from build123d import *

# Parameters (mm, degrees)
F0_R     = 15.24
F0_R_2   = 12.7
F0_R_3   = 11.43
F1_DEPTH = 19.05
F0_R_4   = 1.27
F0_R_5   = 4.8718647292
F2_DEPTH = 12.7
F3_DEPTH = 6.35
F5_DEPTH = 7.62


# Not quite as in the source:
# - a feature of the source that left no trace in its solid (it failed there, or was rolled back) is left out
# - the program builds the solid bodies; features that only make, move or delete a surface that nothing else refers to are left out


with BuildPart() as f1:
    # F0 (on Front) → F1 (new body)
    with BuildSketch(Plane.XZ):
        Circle(F0_R)
        Circle(F0_R_2, mode=Mode.SUBTRACT)
        Circle(F0_R_2)
        Circle(F0_R_3, mode=Mode.SUBTRACT)
    extrude(amount=F1_DEPTH)

    # F0 (on Front) → F2 (join)
    with BuildSketch(Plane.XZ):
        Circle(F0_R_3)
        with Locations((-6.35, -3.6661742094)):
            Circle(F0_R_4, mode=Mode.SUBTRACT)
        with Locations((0, -7.3323484187)):
            Circle(F0_R_4, mode=Mode.SUBTRACT)
        with Locations((6.35, -3.6661742094)):
            Circle(F0_R_4, mode=Mode.SUBTRACT)
        with Locations((-6.35, 3.6661742094)):
            Circle(F0_R_4, mode=Mode.SUBTRACT)
        Circle(F0_R_5, mode=Mode.SUBTRACT)
        with Locations((6.35, 3.6661742094)):
            Circle(F0_R_4, mode=Mode.SUBTRACT)
        with Locations((0, 7.3323484187)):
            Circle(F0_R_4, mode=Mode.SUBTRACT)
    extrude(amount=F2_DEPTH)

    # F0 (on Front) → F3 (join)
    with BuildSketch(Plane.XZ):
        Circle(F0_R_5)
        Polygon((3.175, 1.27), (3.175, -1.27), (1.27, -1.27), (1.27, -3.175), (-1.27, -3.175), (-1.27, -1.27), (-3.175, -1.27), (-3.175, 1.27), (-1.27, 1.27), (-1.27, 3.175), (1.27, 3.175), (1.27, 1.27), align=None, mode=Mode.SUBTRACT)
        with Locations((6.35, 3.6661742094)):
            Circle(F0_R_4)
    extrude(amount=F3_DEPTH)

    # F0 (on Front) + F4 (on face) → F5 (join)
    with BuildSketch(Plane.XZ):
        with Locations((0, 7.3323484187)):
            Circle(F0_R_4)
        with Locations((6.35, -3.6661742094)):
            Circle(F0_R_4)
        with Locations((0, -7.3323484187)):
            Circle(F0_R_4)
        with Locations((-6.35, -3.6661742094)):
            Circle(F0_R_4)
        with Locations((-6.35, 3.6661742094)):
            Circle(F0_R_4)
    with BuildSketch(Plane(origin=(0, 0, 0), x_dir=(-1, 0, 0), z_dir=(0, 1, 0))):
        with BuildLine():
            ThreePointArc((-1.27, 7.3323484187), (0, 6.0623484187), (1.27, 7.3323484187))
            ThreePointArc((1.27, 7.3323484187), (0, 8.6023484187), (-1.27, 7.3323484187))
        make_face()
        with BuildLine():
            ThreePointArc((7.61993774, 3.678749442), (5.715, 4.7660264722), (5.7041406591, 2.5726634816))
            Line((5.7041406591, 2.5726634816), (7.61993774, 3.678749442))
        make_face()
        with BuildLine():
            Line((7.61993774, 3.678749442), (5.7041406591, 2.5726634816))
            ThreePointArc((5.7041406591, 2.5726634816), (6.9795469153, 2.5631915796), (7.62, 3.6661742094))
            ThreePointArc((7.62, 3.6661742094), (7.6199844349, 3.6724619027), (7.61993774, 3.678749442))
        make_face()
        with BuildLine():
            ThreePointArc((-1.27, 12.6363404513), (0, 12.7), (1.27, 12.6363404513))
            Line((1.27, 12.6363404513), (1.27, 15.1869911437))
            ThreePointArc((1.27, 15.1869911437), (0, 15.24), (-1.27, 15.1869911437))
            Line((-1.27, 15.1869911437), (-1.27, 12.6363404513))
        make_face()
        with BuildLine():
            Line((1.27, 15.1869911437), (1.27, 12.6363404513))
            ThreePointArc((1.27, 12.6363404513), (6.0659933949, 11.1576755703), (9.9146853041, 7.9365619333))
            Line((9.9146853041, 7.9365619333), (12.1355541331, 9.2187811496))
            ThreePointArc((12.1355541331, 9.2187811496), (7.3370363933, 13.3576007188), (1.27, 15.1869911437))
        make_face()
        with BuildLine():
            ThreePointArc((-11.4830868745, 5.4248240371), (-10.8829390696, 6.5461161927), (-10.1736532809, 7.6017615668))
            ThreePointArc((-10.1736532809, 7.6017615668), (-6.2510836052, 11.0550420063), (-1.27, 12.6363404513))
            Line((-1.27, 12.6363404513), (-1.27, 15.1869911437))
            ThreePointArc((-1.27, 15.1869911437), (-10.3175287739, -11.2163363002), (15.24, 0))
            ThreePointArc((15.24, 0), (14.7984009497, 3.6421050686), (13.4991956259, 7.0731405651))
            Line((13.4991956259, 7.0731405651), (11.2972745003, 5.8018608105))
            ThreePointArc((11.2972745003, 5.8018608105), (12.344338503, 2.9845111698), (12.7, 0))
            ThreePointArc((12.7, 0), (12.5183628333, -2.1402317572), (11.9786469332, -4.2192437297))
            ThreePointArc((11.9786469332, -4.2192437297), (11.4947402206, -5.4000877087), (10.8947701838, -6.5264065642))
            ThreePointArc((10.8947701838, -6.5264065642), (7.1599884636, -10.4892595163), (2.108859222, -12.5236860701))
            ThreePointArc((2.108859222, -12.5236860701), (0.843104089, -12.6719838816), (-0.431140778, -12.6926796867))
            ThreePointArc((-0.431140778, -12.6926796867), (-5.8966986399, -11.2480640623), (-10.1938394294, -7.5746707973))
            ThreePointArc((-10.1938394294, -7.5746707973), (-10.9002856113, -6.5171906211), (-11.4974295134, -5.3943595157))
            ThreePointArc((-11.4974295134, -5.3943595157), (-12.6999888406, 0.0168359612), (-11.4830868745, 5.4248240371))
        make_face()
        with BuildLine():
            Line((12.1355541331, 9.2187811496), (9.9146853041, 7.9365619333))
            ThreePointArc((9.9146853041, 7.9365619333), (10.6595519093, 6.9039085374), (11.2972745003, 5.8018608105))
            Line((11.2972745003, 5.8018608105), (13.4991956259, 7.0731405651))
            ThreePointArc((13.4991956259, 7.0731405651), (12.8621942988, 8.1744454135), (12.1355541331, 9.2187811496))
        make_face()
        with BuildLine():
            ThreePointArc((7.62, -3.6661742094), (6.5784622338, -2.4168924126), (5.1621968382, -3.2167038))
            Line((5.1621968382, -3.2167038), (7.3331543737, -4.4701067174))
            ThreePointArc((7.3331543737, -4.4701067174), (7.5461408894, -4.0929610094), (7.62, -3.6661742094))
        make_face()
        with BuildLine():
            Line((7.3331543737, -4.4701067174), (5.1621968382, -3.2167038))
            ThreePointArc((5.1621968382, -3.2167038), (5.715, -4.7660264722), (7.3331543737, -4.4701067174))
        make_face()
        with BuildLine():
            ThreePointArc((-5.08, -3.6661742094), (-5.4364655228, -2.7839300487), (-6.305755526, -2.3969451416))
            Line((-6.305755526, -2.3969451416), (-7.4713068529, -3.0698765139))
            ThreePointArc((-7.4713068529, -3.0698765139), (-6.6572786169, -4.8984403541), (-5.08, -3.6661742094))
        make_face()
        with BuildLine():
            Line((-7.4713068529, -3.0698765139), (-6.305755526, -2.3969451416))
            ThreePointArc((-6.305755526, -2.3969451416), (-6.985, -2.5663219465), (-7.4713068529, -3.0698765139))
        make_face()
    extrude(amount=F5_DEPTH, dir=(0, -1, 0))


solid = f1.part
Design review of the part built by this model. Coordinates are the model's own, in mm. A direction names the side the tool comes from. Give positions to 0.01 mm unless a question says otherwise; leave off trailing zeros. Write each loop counter-clockwise with the first axis right and the second up, starting at its lowest first coordinate (ties: lowest second). Pieces come first, ordered by that corner, then holes. Notation, with made-up numbers: M 89,-14 L 126,-14 A28 ccw 126,19 Z; hole C -12.75,62.5 d6. An arc over 180 degrees is marked long. Answer as a JSON object with one key per item and string values. Group by question number.
1) For line 1 along Z through (x, y) = (-6.35, -11.05); line 2 along Z through (x, y) = (1.5, -18); line 3 along X through (y, z) = (-13.5, -4.5), list the stretches that pass through material, from the lowest coordinate up.
2) Tool access review of faces 3 (the face through (0, -3, 3.175)), 4 (the face through (5.41, -10.12, -2.81)), 5 (the face through (0, 0, 4)): name each direction out of +Z, -Z, +X, -X, +Y, -Y from which nothing blocks a thin tool from reaching the whole face with its end or side.
3) We need section C-C (y = -1.5). Give the boundary of the cut face in (x, z) (3 decimals), and give its area (3 significant figures).
4) We need section D-D (y = -12). Give the boundary of the cut face in (x, z), and give its area (3 significant figures).
5) We need section B-B (x = 0). Give the boundary of the cut face in (y, z) (3 decimals), and give its area (3 significant figures).
6) We need section A-A (z = 0). Give the boundary of the cut face in (x, y) (3 decimals).
7) Mouldability with a two-part tool opening along X and no side actions: class faces 1 (the face through (2.2, -19.05, 11.4)), 2 (the face through (-7.29, -10.12, 4.52)) as released by +X, released by -X, zero draft, split by the parting line, or undercut.
8) Clearance check with flat-ended pins moving along their axes: pin 1 Ø1.5 at (y, z) = (-11, -9.5) entering from -X; pin 2 Ø0.6 at (x, y) = (2, -4) entering from +Z; pin 3 Ø8 at (x, y) = (6.5, -16.5) entering from -Z. State where each tip first meets the part, or that it passes through.
Answer key:
{
 "1": {"line 1": "z = -13.85 to -4.94, -2.4 to 2.4, 4.94 to 13.85", "line 2": "z = -15.17 to -11.33, 11.33 to 15.17", "line 3": "x = -14.56 to -10.51, 10.51 to 14.56"},
 "2": {"face 3": "+Y, -Y", "face 4": "-Y", "face 5": "+Z, -Z, +X, -X, +Y"},
 "3": {"outline": "C 0,0 d30.48; hole M -3.175,-1.27 L -1.27,-1.27 L -1.27,-3.175 L 1.27,-3.175 L 1.27,-1.27 L 3.175,-1.27 L 3.175,1.27 L 1.27,1.27 L 1.27,3.175 L -1.27,3.175 L -1.27,1.27 L -3.175,1.27 Z", "area": "704 mm²"},
 "4": {"outline": "C 0,0 d30.48; hole C -6.35,-3.67 d2.54; hole C -6.35,3.67 d2.54; hole C 0,0 d9.74; hole C 0,-7.33 d2.54; hole C 0,7.33 d2.54; hole C 6.35,-3.67 d2.54; hole C 6.35,3.67 d2.54", "area": "625 mm²"},
 "5": {"outline": "M -19.05,-15.24 L 0,-15.24 L 0,-3.175 L -6.35,-3.175 L -6.35,-4.872 L -12.7,-4.872 L -12.7,-6.062 L -7.62,-6.062 L -7.62,-8.602 L -12.7,-8.602 L -12.7,-11.43 L -19.05,-11.43 Z; M -19.05,11.43 L -12.7,11.43 L -12.7,8.602 L -7.62,8.602 L -7.62,6.062 L -12.7,6.062 L -12.7,4.872 L -6.35,4.872 L -6.35,3.175 L 0,3.175 L 0,15.24 L -19.05,15.24 Z", "area": "307 mm²"},
 "6": {"outline": "M -15.24,-19.05 L -11.43,-19.05 L -11.43,-12.7 L -4.872,-12.7 L -4.872,-6.35 L -3.175,-6.35 L -3.175,0 L -15.24,0 Z; M 3.175,-6.35 L 4.872,-6.35 L 4.872,-12.7 L 11.43,-12.7 L 11.43,-19.05 L 15.24,-19.05 L 15.24,0 L 3.175,0 Z"},
 "7": {"face 1": "zero draft", "face 2": "undercut"},
 "8": {"pin 1": "stops at x = -12.48", "pin 2": "stops at z = 15.14", "pin 3": "stops at z = -15.03"}
}
